Part print with two shaded views. Sizes in mm from the minimum x, y, z corner. Round coordinates to 2 decimals unless told otherwise and drop trailing zeros. Write each loop counter-clockwise with the first axis right and the second up, starting at its lowest first coordinate (ties: lowest second). Pieces come first, ordered by that corner, then holes. Notation, with made-up numbers: (30.25, -20.5) -> (44.25, -20.5) arc R10 ccw to (44.25, -12.5) -> close; hole circle Ø3 at (64, -24). An arc over 180 degrees is marked (long way). Answer in a Markdown table with one row per item. Add a question column.
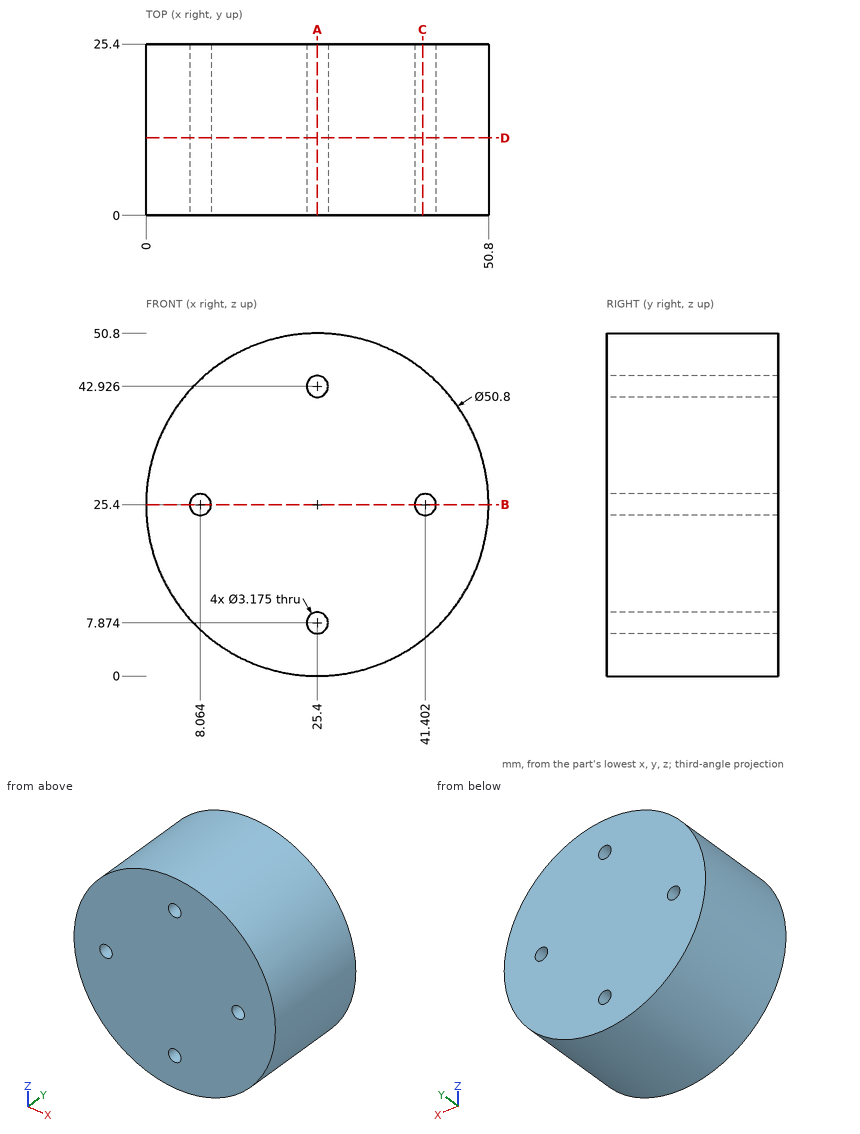
Item 1: Saw through at C-C on x = 41. Give the cut face in (y, z) (1 decimal).
Item 2: Drill centre lines: probe 1 along Z at (x, y) = (25.4, 19.25); probe 2 along X at (y, z) = (6.5, 25) (1 decimal); probe 3 along X at (y, z) = (22.5, 43.5). Where is each one in solid material? Low to high.
Item 3: Saw through at B-B on z = 25.4. Give the cut face in (x, y) (1 decimal), then the cut area to 3 significant figures.
Item 4: Saw through at A-A on x = 25.4. Give the cut face in (y, z).
Item 5: Saw through at D-D on y = 11.5. Give the cut face in (x, z) (1 decimal).
Item 6: Pin check, flat tips, straight feed: pin 1 (4 mm diameter, centred on x = 41.402, z = 25.4, fed in from -Y); pin 2 (5 mm diameter, centred on x = 41, y = 18.5, fed in from +Z); pin 3 (3 mm diameter, centred on x = 45.5, y = 4, fed in from -Z); pin 4 (6 mm diameter, centred on y = 22, z = 30, fed in from +X). Stop position of each tip, or through.
Recorded:
| question | item | result |
|---|---|---|
| 1 | outline | (0, 5.4) -> (25.4, 5.4) -> (25.4, 23.9) -> (0, 23.9) -> close; (0, 26.9) -> (25.4, 26.9) -> (25.4, 45.4) -> (0, 45.4) -> close |
| 2 | probe 1 | 0 to 6.29, 9.46 to 41.34, 44.51 to 50.8 |
| 2 | probe 2 | 0 to 6.5, 9.6 to 39.9, 42.9 to 50.8 |
| 2 | probe 3 | 7.58 to 23.92, 26.88 to 43.22 |
| 3 | outline | (0, 0) -> (6.5, 0) -> (6.5, 25.4) -> (0, 25.4) -> close; (9.7, 0) -> (39.8, 0) -> (39.8, 25.4) -> (9.7, 25.4) -> close; (43, 0) -> (50.8, 0) -> (50.8, 25.4) -> (43, 25.4) -> close |
| 3 | area | 1,130 mm2 |
| 4 | outline | (0, 0) -> (25.4, 0) -> (25.4, 6.29) -> (0, 6.29) -> close; (0, 9.46) -> (25.4, 9.46) -> (25.4, 41.34) -> (0, 41.34) -> close; (0, 44.51) -> (25.4, 44.51) -> (25.4, 50.8) -> (0, 50.8) -> close |
| 5 | outline | circle Ø50.8 at (25.4, 25.4); hole circle Ø3.2 at (8.1, 25.4); hole circle Ø3.2 at (25.4, 7.9); hole circle Ø3.2 at (25.4, 42.9); hole circle Ø3.2 at (41.4, 25.4) |
| 6 | pin 1 | y = 0 |
| 6 | pin 2 | z = 47.16 |
| 6 | pin 3 | z = 8.1 |
| 6 | pin 4 | x = 50.75 |
